The model under review builds one solid part; all positions refer to its coordinate system, in mm. A direction names the side the tool comes from. Coordinates: 2 decimals unless noted, no trailing zeros. Order: outer loops, then holes, each group sorted by start corner. A loop starts at its lowest first (then second) coordinate and runs counter-clockwise, first axis right, second up.
```python
from build123d import *

# Parameters (mm, degrees)
SKETCH_1_W           = 78
SKETCH_1_H           = 78
EXTRUDE_1_DEPTH      = 5.5
SKETCH_2_W           = 78
SKETCH_2_H           = 78
SKETCH_2_W_2         = 74
SKETCH_2_H_2         = 74
SKETCH_2_W_3         = 5
SKETCH_2_H_3         = 5
EXTRUDE_2_DEPTH      = 13
FILLET_1_R           = 1.5
FILLET_2_R           = 3.5
CUT_EXTRUDE_1_DEPTH  = 1
CUT_EXTRUDE_2_DEPTH  = 2.5
SKETCH_5_R           = 1
CUT_EXTRUDE_3_DEPTH  = 58.864064842
CHAMFER_1_SIZE       = 0.5
SKETCH_6_W           = 55
SKETCH_6_H           = 2
SKETCH_6_W_2         = 45
SKETCH_6_H_2         = 55
SKETCH_6_W_3         = 8
SKETCH_6_H_3         = 42
CUT_EXTRUDE_4_DEPTH  = 58.15767665
EXTRUDE_3_DEPTH      = 1
EXTRUDE_3_DEPTH_BACK = 2
SKETCH_7_W           = 49
SKETCH_7_H           = 1.5
SKETCH_7_W_2         = 1.5
SKETCH_7_H_2         = 49


with BuildPart() as part:
    # 草图1 → 凸台-拉伸1 (new body)
    with BuildSketch(Plane.XY):
        Rectangle(SKETCH_1_W, SKETCH_1_H)
    extrude(amount=EXTRUDE_1_DEPTH)

    # 草图2 → 凸台-拉伸2 (add)
    # profile 1 of 5: a face of its own
    with BuildSketch(Plane.XY.offset(5.5)):
        Rectangle(SKETCH_2_W, SKETCH_2_H)
        Rectangle(SKETCH_2_W_2, SKETCH_2_H_2, mode=Mode.SUBTRACT)
    # profile 2 of 5: a face of its own
    with BuildSketch(Plane.XY.offset(5.5)):
        with Locations((-34.5, 34.5)):
            Rectangle(SKETCH_2_W_3, SKETCH_2_H_3)
    # profile 3 of 5: a face of its own
    with BuildSketch(Plane.XY.offset(5.5)):
        with Locations((34.5, 34.5)):
            Rectangle(SKETCH_2_W_3, SKETCH_2_H_3)
    # profile 4 of 5: a face of its own
    with BuildSketch(Plane.XY.offset(5.5)):
        with Locations((34.5, -34.5)):
            Rectangle(SKETCH_2_W_3, SKETCH_2_H_3)
    # profile 5 of 5: a face of its own
    with BuildSketch(Plane.XY.offset(5.5)):
        with Locations((-34.5, -34.5)):
            Rectangle(SKETCH_2_W_3, SKETCH_2_H_3)
    extrude(amount=EXTRUDE_2_DEPTH)

    # 圆角1
    fillet_1_edges = [part.edges().sort_by_distance(p)[0] for p in [
        (-37, -32, 12),
        (-37, 32, 12),
        (-32, 32, 12),
        (-32, 37, 12),
        (32, 37, 12),
        (32, 32, 12),
        (37, 32, 12),
        (37, -32, 12),
        (32, -32, 12),
        (32, -37, 12),
        (-32, -37, 12),
        (-32, -32, 12),
    ]]
    fillet(fillet_1_edges, radius=FILLET_1_R)

    # 圆角2
    fillet_2_edges = [part.edges().sort_by_distance(p)[0] for p in [
        (39, -39, 9.25),
        (-39, -39, 9.25),
        (-39, 39, 9.25),
        (39, 39, 9.25),
    ]]
    fillet(fillet_2_edges, radius=FILLET_2_R)

    # 草图3 → 切除-拉伸1 (cut)
    with BuildSketch(Plane(origin=(0, 0, 0), x_dir=(-1, 0, 0), z_dir=(0, 0, -1))):
        with BuildLine():
            Line((37.5, -35.5), (37.5, 35.5))
            ThreePointArc((37.5, 35.5), (36.914213562, 36.914213562), (35.5, 37.5))
            Line((35.5, 37.5), (-35.5, 37.5))
            ThreePointArc((-35.5, 37.5), (-36.914213562, 36.914213562), (-37.5, 35.5))
            Line((-37.5, 35.5), (-37.5, -35.5))
            ThreePointArc((-37.5, -35.5), (-36.914213562, -36.914213562), (-35.5, -37.5))
            Line((-35.5, -37.5), (35.5, -37.5))
            ThreePointArc((35.5, -37.5), (36.914213562, -36.914213562), (37.5, -35.5))
        make_face()
    extrude(amount=-CUT_EXTRUDE_1_DEPTH, mode=Mode.SUBTRACT)

    # 草图4 → 切除-拉伸2 (cut)
    with BuildSketch(Plane(origin=(0, 0, 1), x_dir=(-1, 0, 0), z_dir=(0, 0, -1))):
        Polygon((27.5, 37.5), (-27.5, 37.5), (-27.5, 36.85), (-32.95, 36.85), (-32.95, -33), (32.95, -33), (32.95, 36.85), (27.5, 36.85), align=None)
    extrude(amount=-CUT_EXTRUDE_2_DEPTH, mode=Mode.SUBTRACT)

    # 草图5 → 切除-拉伸3 (cut, through all)
    with BuildSketch(Plane(origin=(0, 0, 1), x_dir=(-1, 0, 0), z_dir=(0, 0, -1))):
        with Locations((-34.5, 34.5)):
            Circle(SKETCH_5_R)
        with Locations((34.5, 34.5)):
            Circle(SKETCH_5_R)
        with Locations((34.5, -34.5)):
            Circle(SKETCH_5_R)
        with Locations((-34.5, -34.5)):
            Circle(SKETCH_5_R)
    extrude(amount=-CUT_EXTRUDE_3_DEPTH, mode=Mode.SUBTRACT)

    # 倒角1
    chamfer_1_edges = [part.edges().sort_by_distance(p)[0] for p in [
        (-39, 0, 0),
        (39, 0, 0),
        (0, -39, 0),
        (0, 39, 0),
        (-37.974873734, -37.974873734, 0),
        (37.974873734, -37.974873734, 0),
        (37.974873734, 37.974873734, 0),
        (-37.974873734, 37.974873734, 0),
    ]]
    chamfer(chamfer_1_edges, length=CHAMFER_1_SIZE)

    # 草图6 → 切除-拉伸4 (cut, through all)
    with BuildSketch(Plane(origin=(0, 0, 3.5), x_dir=(-1, 0, 0), z_dir=(0, 0, -1))):
        with Locations((0, 36.5)):
            Rectangle(SKETCH_6_W, SKETCH_6_H)
        with Locations((0, 2)):
            Rectangle(SKETCH_6_W_2, SKETCH_6_H_2)
        with Locations((30, 6.1)):
            Rectangle(SKETCH_6_W_3, SKETCH_6_H_3)
    extrude(amount=-CUT_EXTRUDE_4_DEPTH, mode=Mode.SUBTRACT)

    # 草图7 → 凸台-拉伸3 (add, two sides: drawn at the far end of the back side and taken through both)
    with BuildSketch(Plane.XY.offset(18.5).offset(-EXTRUDE_3_DEPTH_BACK)):
        with Locations((0, 36.75)):
            Rectangle(SKETCH_7_W, SKETCH_7_H)
        with Locations((-36.75, 0)):
            Rectangle(SKETCH_7_W_2, SKETCH_7_H_2)
        with Locations((0, -36.75)):
            Rectangle(SKETCH_7_W, SKETCH_7_H)
        with Locations((36.75, 0)):
            Rectangle(SKETCH_7_W_2, SKETCH_7_H_2)
    extrude(amount=EXTRUDE_3_DEPTH + EXTRUDE_3_DEPTH_BACK)


solid = part.part
```
(1) Wall thickness on probe 1 along Y at (x, z) = (34.5, 13.5); probe 2 along Y at (x, z) = (-10, 8.5); probe 3 along Y at (x, z) = (34.5, 4.75): over which ranges is each line inside the solid? List them lowest first.
A:
probe 1: y = -39 to -35.5, -33.5 to -32, 32 to 33.5, 35.5 to 39
probe 2: y = -39 to -37, 37.5 to 39
probe 3: y = -39 to -35.5, -33.5 to 33.5, 35.5 to 39
(2) Draft analysis for pull direction Y (two halves, no side actions). For faces 4 (the face through (38, 37.95, 9.37)), 5 (the face through (29, 37, 12)), 6 (the face through (-39, 0, 9)), state which applies: released by +Y, released by -Y, zero draft, split by the parting line, or undercut.
A:
face 4: released by +Y
face 5: undercut
face 6: zero draft
(3) We need section A-A, the plane y = 34.5. Write out the cut boundary in (x, z), and give its area (3 significant figures).
A:
outline: (-39, 0.5) - (-38.5, 0) - (-37.5, 0) - (-37.5, 1) - (-35.5, 1) - (-35.5, 18.5) - (-39, 18.5) - close; (-33.5, 1) - (-32.95, 1) - (-32.95, 3.5) - (32.95, 3.5) - (32.95, 1) - (33.5, 1) - (33.5, 18.5) - (32, 18.5) - (32, 5.5) - (-32, 5.5) - (-32, 18.5) - (-33.5, 18.5) - close; (35.5, 1) - (37.5, 1) - (37.5, 0) - (38.5, 0) - (39, 0.5) - (39, 18.5) - (35.5, 18.5) - close
area: 301 mm2
(4) We need section C-C, the plane y = -34.5. Write out the cut boundary in (x, z), and give its area (3 significant figures).
A:
outline: (-39, 0.5) - (-38.5, 0) - (-37.5, 0) - (-37.5, 1) - (-35.5, 1) - (-35.5, 18.5) - (-39, 18.5) - close; (-33.5, 1) - (33.5, 1) - (33.5, 18.5) - (32, 18.5) - (32, 5.5) - (-32, 5.5) - (-32, 18.5) - (-33.5, 18.5) - close; (35.5, 1) - (37.5, 1) - (37.5, 0) - (38.5, 0) - (39, 0.5) - (39, 18.5) - (35.5, 18.5) - close
area: 466 mm2
(5) We need section B-B, the plane x = 2. Write out the cut boundary in (y, z).
A:
outline: (-39, 0.5) - (-38.5, 0) - (-37.5, 0) - (-37.5, 1) - (-33, 1) - (-33, 3.5) - (-25.5, 3.5) - (-25.5, 5.5) - (-37, 5.5) - (-37, 16.5) - (-36, 16.5) - (-36, 19.5) - (-37.5, 19.5) - (-37.5, 18.5) - (-39, 18.5) - close; (29.5, 3.5) - (35.5, 3.5) - (35.5, 5.5) - (29.5, 5.5) - close; (36, 16.5) - (37.5, 16.5) - (37.5, 0) - (38.5, 0) - (39, 0.5) - (39, 18.5) - (37.5, 18.5) - (37.5, 19.5) - (36, 19.5) - close
(6) For pin 1 Ø6 at (x, y) = (-23, -16) entering from -Z; pin 2 Ø0.8 at (x, y) = (-33.5, 0.5) entering from +Z; pin 3 Ø2.5 at (x, y) = (34.5, -34.5) entering from -Z, all flat-tipped, find the tip position at first contact; note any pin that passes through.
A:
pin 1: stops at z = 3.5
pin 2: stops at z = 3.5
pin 3: stops at z = 1
(7) Machinability: for faces 1 (the face through (30, 36.85, 2)), 2 (the face through (0, 29.5, 4)), 3 (the face through (-35, 32, 12)), which of the approach directions +Z, -Z, +X, -X, +Y, -Y give a long, thin tool a straight path to every point of the face, cutting with its end or side? Answer none if there is none.
A:
face 1: -Z
face 2: +Z, -Z
face 3: +Z
